from build123d import *

# Parameters (mm, degrees)
F0_W        = 53.4896697645
F0_H        = 50
F1_DEPTH    = 50
F2_T1_DEPTH = 204.300979278


# Not quite as in the source:
# - a fillet or chamfer that OpenCascade refuses, or shapes differently, is made with other operations: its cross-section is extruded or revolved along the edge and cut away or added


with BuildPart() as f1:
    # F0 (on Front) → F1 (new body)
    with BuildSketch(Plane.XZ):
        with Locations((26.7448348823, 25)):
            Rectangle(F0_W, F0_H)
    extrude(amount=F1_DEPTH)

    # F2: chamfer of 30 on 2 edges, made by hand

    # F2_s2 → F2_t1 (cut)
    with BuildSketch(Plane.XZ.offset(-77.150489639)):
        Polygon((53.4896697645, 20), (23.4896697645, 50), (53.4896697645, 50), align=None)
        Polygon((0, 20), (30, 50), (0, 50), align=None)
    extrude(amount=F2_T1_DEPTH, mode=Mode.SUBTRACT)


solid = f1.part
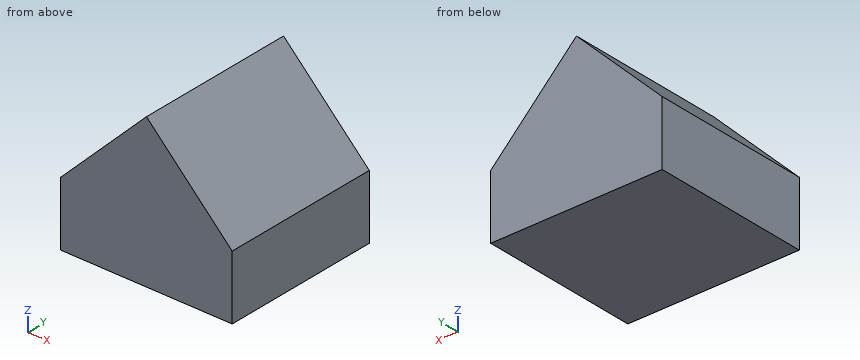
Check sheet for the modelled part. Datum: model origin and axes. Units: mm. Give positions to 0.01 mm unless a question says otherwise; leave off trailing zeros. Loops run counter-clockwise (first coordinate to the right, second up) from the corner with the lowest first, then second, coordinate; pieces in that order, holes last. Notation, with made-up numbers: M 41,10.5 L 75,10.5 A23 cw 75,40.5 Z; hole C -27.75,-7.75 d5. An arc over 180 degrees is marked long. Return JSON: item names as keys, results as strings. Group by question number.
1. Go/stop test with a flat-tipped pin: pin 1 (12 mm diameter, centred on x = 43.5, y = -14.5, fed in from +Z). Record where the tip stops, or that it passes through.
2. Thickness scan on L1, parallel to X at y = -39, z = 30; L2, parallel to Z at x = 50.5, y = -39; L3, parallel to Z at x = 31.5, y = -44.5. Record the ranges inside material, lowest first.
3. Cross-section at B-B on x = 23. Record the boundary of the cut face in (y, z), plus the area to 3 significant figures.
4. Cross-section at C-C on z = 39.5. Record the boundary of the cut face in (x, y).
5. Cross-section at A-A on y = -39. Record the boundary of the cut face in (x, z), plus the area to 3 significant figures.
Return value:
{
 "1": {"pin 1": "z = 35.99"},
 "2": {"L1": "10 to 43.49", "L2": "0 to 22.99", "L3": "0 to 41.99"},
 "3": {"outline": "M -50,0 L 0,0 L 0,43 L -50,43 Z", "area": "2,150 mm^2"},
 "4": {"outline": "M 19.5,-50 L 33.99,-50 L 33.99,0 L 19.5,0 Z"},
 "5": {"outline": "M 0,0 L 53.49,0 L 53.49,20 L 26.74,46.74 L 0,20 Z", "area": "1,790 mm^2"}
}
